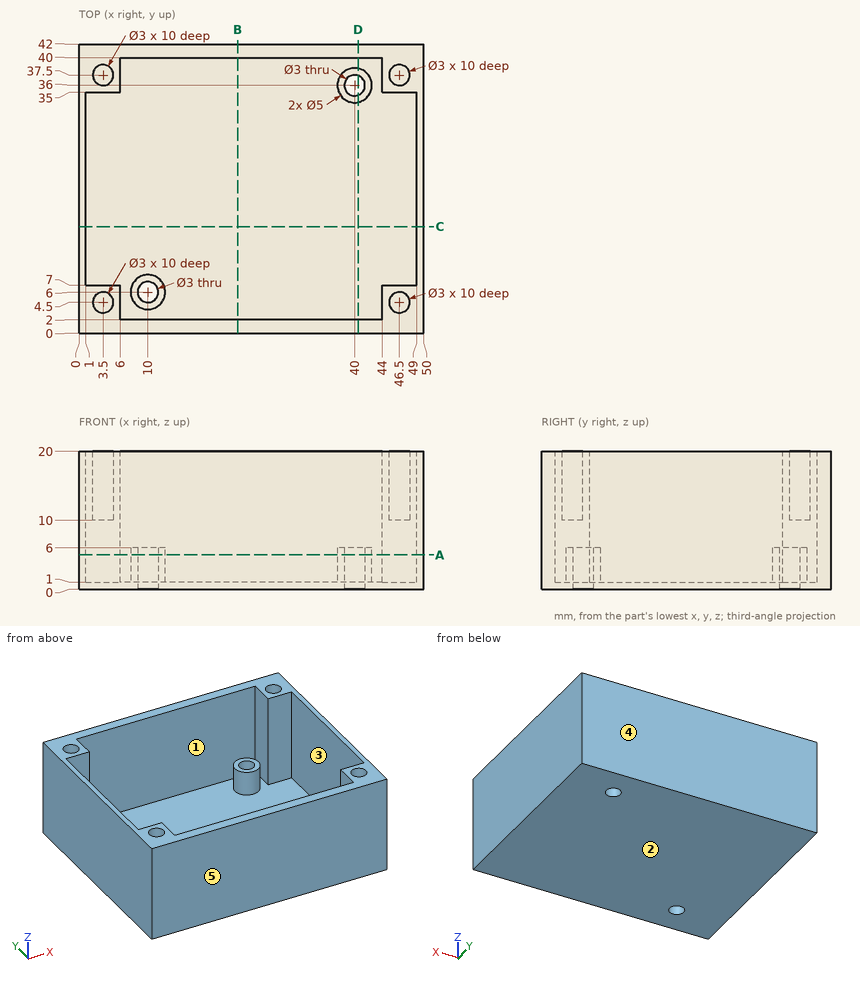
Part print with two shaded views. Sizes in mm from the minimum x, y, z corner. A direction names the side the tool comes from. Round coordinates to 2 decimals unless told otherwise and drop trailing zeros. Write each loop counter-clockwise with the first axis right and the second up, starting at its lowest first coordinate (ties: lowest second). Pieces come first, ordered by that corner, then holes. Notation, with made-up numbers: (59.5, 9.25) -> (75.5, 9.25) arc R29 ccw to (75.5, 42.25) -> close; hole circle Ø2 at (61.25, -39). An arc over 180 degrees is marked (long way). Put each result on its own line as item: value.
Item 1: Flat gauge pins, fed straight in: P1, Ø2.5, axis at x = 46.5, y = 37.5, coming from the +Z side; P2, Ø1.5, axis at x = 35.5, y = 32.5, coming from the +Z side; P3, Ø1.5, axis at x = 39, y = 36, coming from the +Z side. Where does each tip first touch, or does it go through?
Here are the results:
P1: stops at z = 10
P2: stops at z = 1
P3: stops at z = 6
Item 2: Tool access for the marked faces 1 and 2: list every direction of +Z, -Z, +X, -X, +Y, -Y with a clear straight run to the whole face (end or side of a thin tool).
Here are the results:
face 1: +Z
face 2: -Z, +X, -X, +Y, -Y
Item 3: Slice it at B-B, the plane x = 23. Give the cut face in (y, z).
Here are the results:
outline: (0, 0) -> (42, 0) -> (42, 20) -> (40, 20) -> (40, 1) -> (2, 1) -> (2, 20) -> (0, 20) -> close
Item 4: Slice it at D-D, the plane x = 40.5. Give the cut face in (y, z), plus the area to 3 significant figures.
Here are the results:
outline: (0, 0) -> (34.59, 0) -> (34.59, 6) -> (33.55, 6) -> (33.55, 1) -> (2, 1) -> (2, 20) -> (0, 20) -> close; (37.41, 0) -> (42, 0) -> (42, 20) -> (40, 20) -> (40, 1) -> (38.45, 1) -> (38.45, 6) -> (37.41, 6) -> close
area: 126 mm^2
Item 5: Wall check: probe 1 along Y at (x, z) = (10, 2.5); probe 2 along Y at (x, z) = (46.5, 12.5); probe 3 along X at (y, z) = (34, 2.25). Give the ranges that are in metal, low to high. Write a range as from..to.
Here are the results:
probe 1: y = 0..2, 3.5..4.5, 7.5..8.5, 40..42
probe 2: y = 0..3, 6..7, 35..36, 39..42
probe 3: x = 0..1, 38.5..41.5, 49..50
Item 6: Two-plate mould, pull along Y, no slides. Class the marked faces 3, 4 and 5: pulls with the +Y half, pulls with the -Y half, needs draft (parallel to the pull), parting line crosses it, or undercut.
Here are the results:
face 3: undercut
face 4: pulls with the +Y half
face 5: pulls with the -Y half
Item 7: Slice it at A-A, the plane z = 5. Give the cut face in (x, y).
Here are the results:
outline: (0, 0) -> (50, 0) -> (50, 42) -> (0, 42) -> close; circle Ø5 at (10, 6); circle Ø5 at (40, 36); hole (1, 7) -> (6, 7) -> (6, 2) -> (44, 2) -> (44, 7) -> (49, 7) -> (49, 35) -> (44, 35) -> (44, 40) -> (6, 40) -> (6, 35) -> (1, 35) -> close; hole circle Ø3 at (10, 6); hole circle Ø3 at (40, 36)
Item 8: Slice it at C-C, the plane y = 15.5. Give the cut face in (x, z), plus the area to 3 significant figures.
Here are the results:
outline: (0, 0) -> (50, 0) -> (50, 20) -> (49, 20) -> (49, 1) -> (1, 1) -> (1, 20) -> (0, 20) -> close
area: 88.0 mm^2
